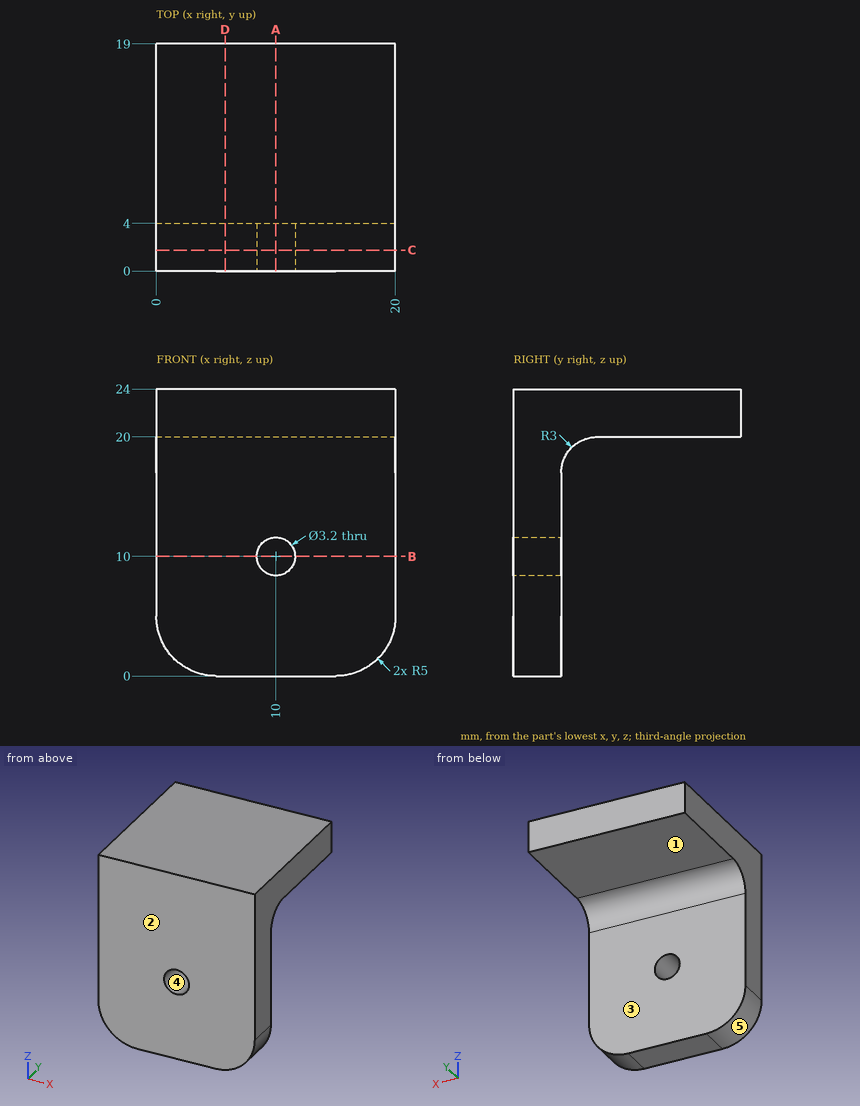
Job drawing, mm, ordinate dimensions from the low corner. One solid piece. A direction names the side the tool comes from. Round coordinates to 2 decimals unless told otherwise and drop trailing zeros. Loops run counter-clockwise (first coordinate to the right, second up) from the corner with the lowest first, then second, coordinate; pieces in that order, holes last.
(1) Cut at D-D (x = 5.75). Give the cut face in (y, z), plus the area to 3 significant figures.
(2) Drop flat-ended pins along their axis: pin 1 (4 mm diameter, centred on x = 4.5, z = 12, fed in from +Y); pin 2 (6 mm diameter, centred on x = 7, y = 13, fed in from -Z). Give the stop position or say it passes through.
(3) Cut at B-B (z = 10). Give the cut face in (x, y), plus the area to 3 significant figures.
(4) Wall check: line 1 along X through (y, z) = (1.9, 10); line 2 along Z through (x, y) = (15.5, 12.25); line 3 along Y through (x, z) = (3.25, 14.75). Give the ranges that are in metal, low to high.
(5) Two-plate mould, pull along X, no slides. Class the marked faces 3, 4 and 5: +X half, -X half, draft (parallel to the pull), parting line (faces both ways), or undercut.
(6) Cut at C-C (y = 1.75). Give the cut face in (x, z).
(7) Which spindle directions (+Z, -Z, +X, -X, +Y, -Y) get a long thin tool onto all of the face, cutting with end or side? Do the marked faces 1 and 2. Say none if no direction does.
(8) Cut at A-A (x = 10). Give the cut face in (y, z), plus the area to 3 significant figures.
Findings below:
1. outline: (0, 0) - (4, 0) - (4, 17) arc R3 cw to (7, 20) - (19, 20) - (19, 24) - (0, 24) - close
1. area: 158 mm2
2. pin 1: stops at y = 4
2. pin 2: stops at z = 20
3. outline: (0, 0) - (8.4, 0) - (8.4, 4) - (0, 4) - close; (11.6, 0) - (20, 0) - (20, 4) - (11.6, 4) - close
3. area: 67.2 mm2
4. line 1: x = 0 to 8.4, 11.6 to 20
4. line 2: z = 20 to 24
4. line 3: y = 0 to 4
5. face 3: draft
5. face 4: undercut
5. face 5: -X half
6. outline: (0, 5) arc R5 ccw to (5, 0) - (15, 0) arc R5 ccw to (20, 5) - (20, 24) - (0, 24) - close; hole circle Ø3.2 at (10, 10)
7. face 1: -Z, +X, -X, +Y
7. face 2: +Z, -Z, +X, -X, -Y
8. outline: (0, 0) - (4, 0) - (4, 8.4) - (0, 8.4) - close; (0, 11.6) - (4, 11.6) - (4, 17) arc R3 cw to (7, 20) - (19, 20) - (19, 24) - (0, 24) - close
8. area: 145 mm2
